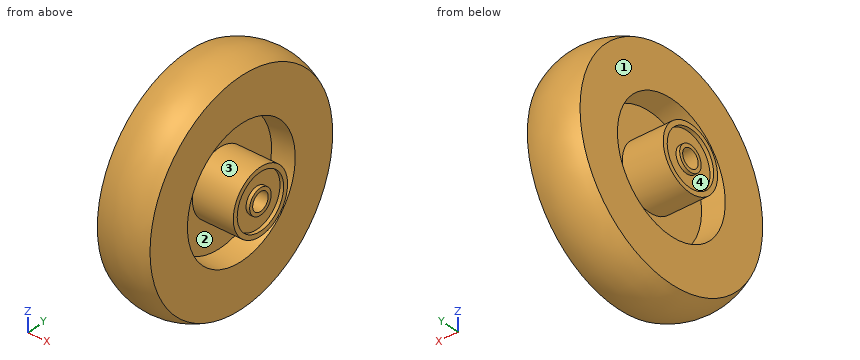
```python
from build123d import *

# Parameters (mm, degrees)
SKETCH2_R          = 19.001809039
SKETCH2_R_2        = 8.788318948
CUT_EXTRUDE1_DEPTH = 2.54
SKETCH3_R          = 6.35
CUT_EXTRUDE2_DEPTH = 64.5


with BuildPart() as part:
    # Sketch1 → Revolve1 (revolve)
    with BuildSketch(Plane(origin=(0, 0, 0), x_dir=(1, 0, 0), z_dir=(0, 1, 0))):
        with BuildLine():
            Line((-31.75, 22.225), (-31.75, 0))
            Line((-31.75, 0), (31.75, 0))
            Line((31.75, 0), (31.75, 22.225))
            Line((31.75, 22.225), (3.175, 22.225))
            Line((3.175, 22.225), (3.175, 42.545))
            Line((3.175, 42.545), (18.415, 44.136059808))
            Line((18.415, 44.136059808), (18.415, 74.737433252))
            ThreePointArc((18.415, 74.737433252), (0, 79.375), (-18.415, 74.737433252))
            Line((-18.415, 74.737433252), (-18.415, 44.136059808))
            Line((-18.415, 44.136059808), (-3.175, 42.545))
            Line((-3.175, 42.545), (-3.175, 22.225))
            Line((-3.175, 22.225), (-31.75, 22.225))
        make_face()
    revolve(axis=Axis((-31.75, 0, 0), (-1, 0, 0)))

    # Sketch2 → Cut-Extrude1 (cut)
    with BuildSketch(Plane(origin=(31.75, 0, 0), x_dir=(0, 0, -1), z_dir=(1, 0, 0))):
        Circle(SKETCH2_R)
        Circle(SKETCH2_R_2, mode=Mode.SUBTRACT)
    cut_extrude1 = extrude(amount=-CUT_EXTRUDE1_DEPTH, mode=Mode.SUBTRACT)

    # Sketch3 → Cut-Extrude2 (cut, through all)
    with BuildSketch(Plane(origin=(31.75, 0, 0), x_dir=(0, 0, -1), z_dir=(1, 0, 0))):
        Circle(SKETCH3_R)
    extrude(amount=-CUT_EXTRUDE2_DEPTH, mode=Mode.SUBTRACT)

    # Mirror3: Cut-Extrude1 across plane
    add(cut_extrude1.mirror(Plane(origin=(0, 0, 0), x_dir=(0, 0, 1), z_dir=(1, 0, 0))), mode=Mode.SUBTRACT)


solid = part.part
```
For this review, take the finished solid that the model builds, in its own axes (mm). Face numbers are marked on the shaded views. A direction names the side the tool comes from. Coordinates: 2 decimals unless noted, no trailing zeros. Loops run counter-clockwise (first coordinate to the right, second up) from the corner with the lowest first, then second, coordinate; pieces in that order, holes last.
1. Insertion check: P1, Ø1.5, axis at y = 11.5, z = 27, coming from the +X side (3 decimals); P2, Ø12, axis at y = -43.5, z = -34, coming from the -X side (3 decimals); P3, Ø6, axis at x = -16, z = -22.5, coming from the -Y side; P4, Ø7.5, axis at y = 0, z = 0, coming from the -X side. Each pin has a flat end and moves straight along its axis. Give the tip position at first contact, or say it passes through.
2. Mouldability with a two-part tool opening along Y and no side actions: class the marked faces 1 and 2 as +Y half, -Y half, draft (parallel to the pull), parting line (faces both ways), or undercut.
3. For line 1 (Y direction, x = 30.9, z = 0) (3 decimals); line 2 (Y direction, x = -17.5, z = 3); line 3 (Y direction, x = 29, z = 0) (3 decimals), list the stretches that pass through material, from the lowest coordinate up.
4. Add section B-B, the plane x = -7.5. Give the boundary of the cut face in (y, z) (3 decimals).
5. Add section A-A, the plane x = 12.5. Give the boundary of the cut face in (y, z) (3 decimals).
6. For the marked faces 3 and 4, list the 3-axis set-ups (+Z, -Z, +X, -X, +Y, -Y) from which the entire face can be reached by the end or side of a thin tool; tool diameter is ignored.
Result:
1. P1: stops at x = 3.175
1. P2: stops at x = -18.415
1. P3: stops at y = -74.08
1. P4: passes through
2. face 1: draft
2. face 2: undercut
3. line 1: y = -22.225 to -19.002, -8.788 to -6.35, 6.35 to 8.788, 19.002 to 22.225
3. line 2: y = -75.15 to -43.94, -22.02 to -5.6, 5.6 to 22.02, 43.94 to 75.15
3. line 3: y = -22.225 to -6.35, 6.35 to 22.225
4. outline: circle Ø157.29 at (0, 0); circle Ø44.45 at (0, 0); hole circle Ø85.993 at (0, 0); hole circle Ø12.7 at (0, 0)
5. outline: circle Ø154.622 at (0, 0); circle Ø44.45 at (0, 0); hole circle Ø87.037 at (0, 0); hole circle Ø12.7 at (0, 0)
6. face 3: +X
6. face 4: -X
